Drawing for the job (mm, zero at the part's lowest x, y, z). A direction names the side the tool comes from. Give positions to 0.01 mm unless a question says otherwise; leave off trailing zeros. Write each loop counter-clockwise with the first axis right and the second up, starting at its lowest first coordinate (ties: lowest second). Pieces come first, ordered by that corner, then holes.
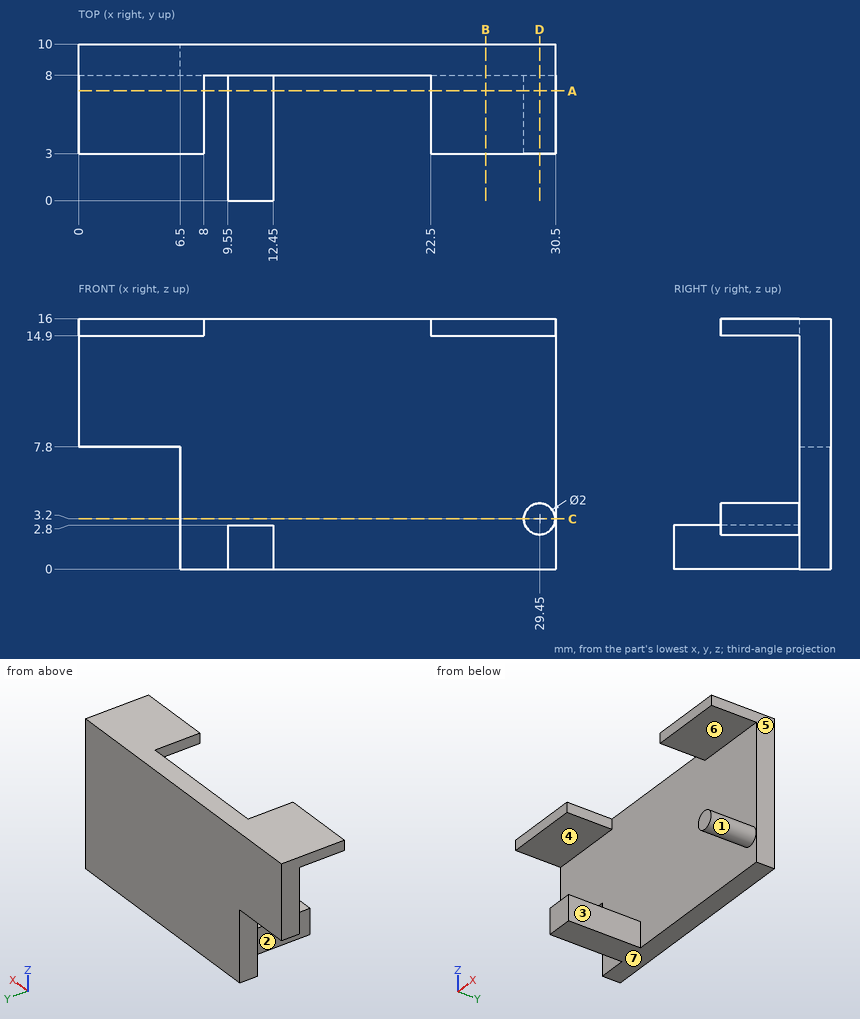
1. Pull direction Z, two halves, no side cores. Call the marked faces 5, 6 and 7: +Z half, -Z half, draft (parallel to the pull), parting line (faces both ways), or undercut.
Calculated:
face 5: draft
face 6: undercut
face 7: -Z half
2. Pin check, flat tips, straight feed: P1, Ø5, axis at x = 12.5, z = 4.5, coming from the -Y side; P2, Ø0.6, axis at x = 29, z = 2.5, coming from the -Y side; P3, Ø2, axis at y = 9, z = 2.5, coming from the -X side; P4, Ø5, axis at y = 5, z = 11, coming from the -X side. Stop position of each tip, or through.
Calculated:
P1: stops at y = 0
P2: stops at y = 3
P3: stops at x = 6.5
P4: passes through
3. Probe probe 1 along Z at (x, y) = (23.5, 6); probe 2 along Y at (x, z) = (8, 3.5); probe 3 along X at (y, z) = (0.5, 1). List the from-to ranges inside material, lowest first.
Calculated:
probe 1: z = 14.9 to 16
probe 2: y = 8 to 10
probe 3: x = 9.55 to 12.45
4. Slice it at A-A, the plane y = 7. Write the cut outline in (x, z), and give its area (3 significant figures).
Calculated:
outline: (0, 14.9) - (8, 14.9) - (8, 16) - (0, 16) - close; (9.55, 0) - (12.45, 0) - (12.45, 2.8) - (9.55, 2.8) - close; (22.5, 14.9) - (30.5, 14.9) - (30.5, 16) - (22.5, 16) - close; circle Ø2 at (29.45, 3.2)
area: 28.9 mm2
5. Slice it at C-C, the plane z = 3.2. Write the cut outline in (x, y).
Calculated:
outline: (6.5, 8) - (28.45, 8) - (28.45, 3) - (30.45, 3) - (30.45, 8) - (30.5, 8) - (30.5, 10) - (6.5, 10) - close
6. Slice it at D-D, the plane x = 29.45. Write the cut outline in (y, z), and give its area (3 significant figures).
Calculated:
outline: (3, 2.2) - (8, 2.2) - (8, 0) - (10, 0) - (10, 16) - (3, 16) - (3, 14.9) - (8, 14.9) - (8, 4.2) - (3, 4.2) - close
area: 47.5 mm2
7. Which spindle directions (+Z, -Z, +X, -X, +Y, -Y) get a long thin tool onto all of the face, cutting with end or side? Do the marked faces 1, 2, 3 and 4. Say none if no direction does.
Calculated:
face 1: -Y
face 2: +Z, -Z, -X, -Y
face 3: +Z, -Z, -Y
face 4: -Z, +X, -X, -Y
8. Slice it at B-B, the plane x = 26. Write the cut outline in (y, z).
Calculated:
outline: (3, 14.9) - (8, 14.9) - (8, 0) - (10, 0) - (10, 16) - (3, 16) - close
